Verification items for the finished model (mm, model axes). Face numbers are marked on the shaded views. A direction names the side the tool comes from. Round coordinates to 2 decimals unless told otherwise and drop trailing zeros. Write each loop counter-clockwise with the first axis right and the second up, starting at its lowest first coordinate (ties: lowest second). Pieces come first, ordered by that corner, then holes. Notation, with made-up numbers: M 60,30 L 83,30 A20 cw 83,49 Z; hole C -13,71.25 d1. An arc over 180 degrees is marked long. Answer in a Markdown table with one row per item. Add a question column.
1. Sectioned sample at A-A on x = 6. Record the cut outline in (y, z).
2. Sectioned sample at D-D on x = 31. Record the cut outline in (y, z).
3. Sectioned sample at B-B on z = -25. Record the cut outline in (x, y).
4. Sectioned sample at C-C on y = -15. Record the cut outline in (x, z), plus the area to 3 significant figures.
5. Material ranges on probe 1 along X at (y, z) = (-15, -0.5); probe 2 along X at (y, z) = (-1.5, 18); probe 3 along Z at (x, y) = (-3.5, -14.5), recorded low to high.
6. Go/stop test with flat-tipped pins: pin 1 Ø6 at (x, z) = (-3.5, 10) entering from -Y; pin 2 Ø15 at (x, y) = (9, 8.5) entering from +Z; pin 3 Ø8 at (y, z) = (-12, -3) entering from +X; pin 4 Ø4 at (y, z) = (3, 30) entering from +X. Record where each tip stops, or that it passes through.
7. Set-up check for the marked faces 1, 2 and 3: record each of +Z, -Z, +X, -X, +Y, -Y from which the full face is reachable in a straight line by a thin tool's end or side.
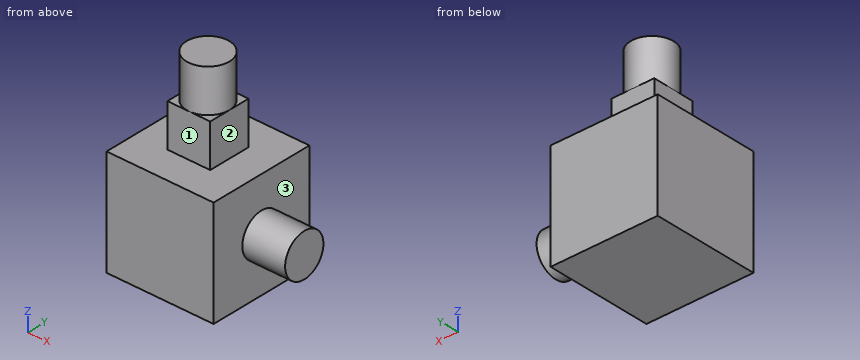
Autodesk Inventor part; units mm, degrees
ref_plane "YZ Plane" through (0, 0, 0) normal (1, 0, 0) x (0, 1, 0)
ref_plane "XZ Plane" through (0, 0, 0) normal (0, 1, 0) x (-1, 0, 0)
ref_plane "XY Plane" through (0, 0, 0) normal (0, 0, 1) x (1, 0, 0)
sketch "Sketch1" plane through (0, 0, 0) normal (0, 0, 1) x (1, 0, 0)
  line L0 (-25, 25) -> (25, 25)
  line L1 (25, 25) -> (25, -25)
  line L2 (25, -25) -> (-25, -25)
  line L3 (-25, -25) -> (-25, 25)
  point P0 (0, 0)
  point P1 (-25, 0)
  point P2 (0, 25)
  dimension "d0" = 50
  dimension "d1" = 50
extrude "Extrusion1" add sketch "Sketch1" against normal blind 50
sketch "Sketch2" plane through (0, 0, 0) normal (0, 0, 1) x (1, 0, 0)
  line L0 (-10, 10) -> (10, 10)
  line L1 (10, 10) -> (10, -10)
  line L2 (10, -10) -> (-10, -10)
  line L3 (-10, -10) -> (-10, 10)
  point P0 (0, 0)
  point P1 (-10, 0)
  point P2 (0, 10)
  dimension "d4" = 20
  dimension "d5" = 20
extrude "Extrusion2" add sketch "Sketch2" along normal blind 20
sketch "Sketch3" plane through (0, 0, 20) normal (0, 0, 1) x (1, 0, 0)
  line L0 (10, 10) -> (10, -10)
  circle A0 centre (0, 0) radius 10
extrude "Extrusion3" add sketch "Sketch3" along normal blind 20
sketch "Sketch4" plane through (25, -25, 0) normal (1, 0, 0) x (0, 0, -1)
  line L0 (50, 0) -> (50, 50)
  line L1 (0, 50) -> (50, 50)
  circle A0 centre (25, 25) radius 10
  point P0 (0, 25)
  point P1 (50, 25)
  point P2 (25, 50)
  dimension "d10" = 20
extrude "Extrusion4" add sketch "Sketch4" along normal blind 20
properties part number "cubo 2"
Geometry check:
| question | item | result |
|---|---|---|
| 1 | outline | M -25,-50 L 25,-50 L 25,0 L 10,0 L 10,20 L 8,20 L 8,40 L -8,40 L -8,20 L -10,20 L -10,0 L -25,0 Z |
| 2 | outline | C 0,-25 d20 |
| 3 | outline | M -25,-25 L 25,-25 L 25,-10 L 45,-10 L 45,10 L 25,10 L 25,25 L -25,25 Z |
| 4 | outline | M -25,-50 L 25,-50 L 25,0 L -25,0 Z |
| 4 | area | 2,500 mm2 |
| 5 | probe 1 | x = -25 to 25 |
| 5 | probe 2 | x = -10 to 10 |
| 5 | probe 3 | z = -50 to 0 |
| 6 | pin 1 | stops at y = -10 |
| 6 | pin 2 | stops at z = 40 |
| 6 | pin 3 | stops at x = 25 |
| 6 | pin 4 | stops at x = 9.95 |
| 7 | face 1 | +Z, +X, -X, -Y |
| 7 | face 2 | +Z, +X, +Y, -Y |
| 7 | face 3 | +X |
